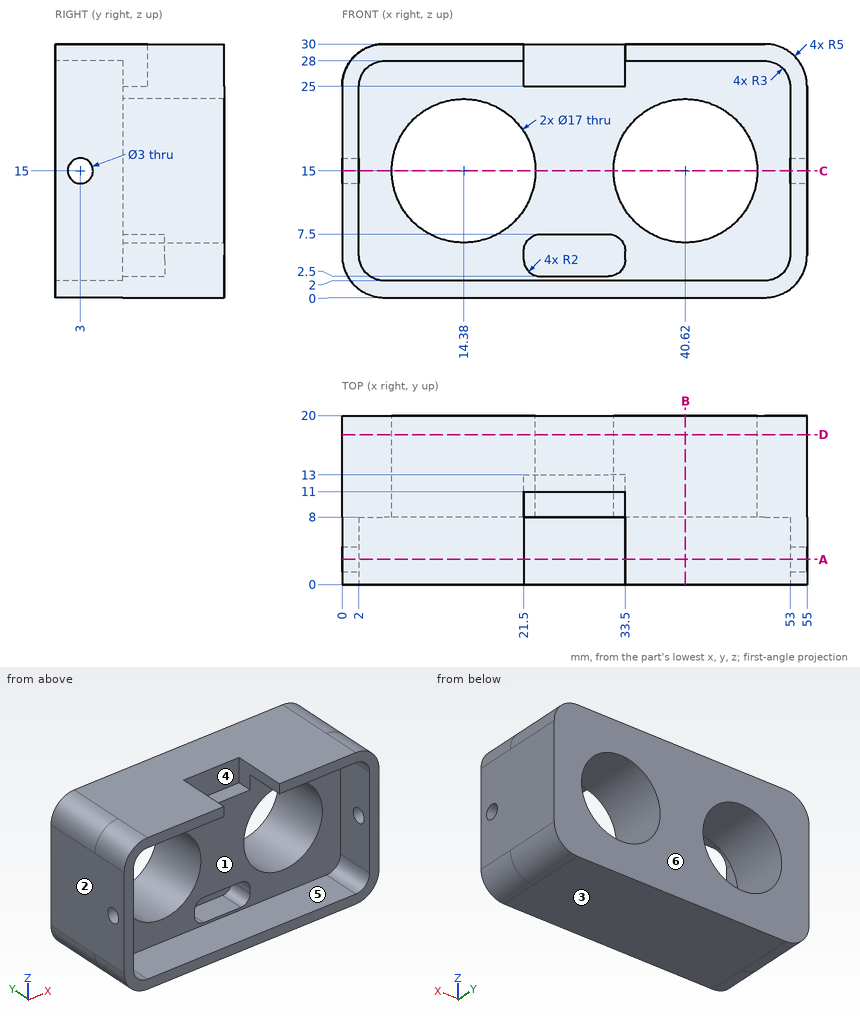
Drawing for the job (mm, zero at the part's lowest x, y, z). A direction names the side the tool comes from. Round coordinates to 2 decimals unless told otherwise and drop trailing zeros. Write each loop counter-clockwise with the first axis right and the second up, starting at its lowest first coordinate (ties: lowest second). Pieces come first, ordered by that corner, then holes. Notation, with made-up numbers: M 42,-9.5 L 72,-9.5 A30 cw 72,13.5 Z; hole C -39.5,85.5 d7. An arc over 180 degrees is marked long. Answer as a JSON object with one key per item and string values. Group by question number.
(1) Cut at D-D (y = 17.75). Give the cut face in (x, z).
(2) Which spindle directions (+Z, -Z, +X, -X, +Y, -Y) get a long thin tool onto all of the face, cutting with end or side? Do the marked faces 4, 5 and 6. Say none if no direction does.
(3) Mould opens along Z. For the marked faces 1, 2 and 3 say: pulls with the +Z half, pulls with the -Z half, needs draft (parallel to the pull), parting line crosses it, or undercut.
(4) Cut at B-B (x = 40.62). Give the cut face in (y, z).
(5) Flat gauge pins, fed straight in: pin 1 (1.5 mm diameter, centred on x = 28.5, z = 6, fed in from -Y); pin 2 (6 mm diameter, centred on x = 22.5, z = 14, fed in from -Y); pin 3 (2.5 mm diameter, centred on x = 26, y = 9.5, fed in from +Z); pin 4 (15.5 mm diameter, centred on x = 40.62, z = 15, fed in from -Y). Where does each tip first touch, or does it go through?
(6) Cut at C-C (z = 15). Give the cut face in (x, y), and give its area (3 significant figures).
(7) Drill centre lines: L1, parallel to X at y = 2, z = 7.5; L2, parallel to X at y = 11.5, z = 15; L3, parallel to X at y = 17.25, z = 14. Where is each one in solid material? Low to high.
(8) Cut at A-A (y = 3). Give the cut face in (x, z), and give its area (3 significant figures).
Responses:
{
 "1": {"outline": "M 0,5 A5 ccw 5,0 L 50,0 A5 ccw 55,5 L 55,25 A5 ccw 50,30 L 5,30 A5 ccw 0,25 Z; hole C 14.38,15 d17; hole C 40.62,15 d17"},
 "2": {"face 4": "+Z, -Y", "face 5": "-Y", "face 6": "+Z, -Z, +X, -X, +Y"},
 "3": {"face 1": "undercut", "face 2": "needs draft", "face 3": "pulls with the -Z half"},
 "4": {"outline": "M 0,0 L 20,0 L 20,6.5 L 8,6.5 L 8,2 L 0,2 Z; M 0,28 L 8,28 L 8,23.5 L 20,23.5 L 20,30 L 0,30 Z"},
 "5": {"pin 1": "stops at y = 13", "pin 2": "stops at y = 8", "pin 3": "stops at z = 25", "pin 4": "passes through"},
 "6": {"outline": "M 0,0 L 2,0 L 2,1.5 L 0,1.5 Z; M 0,4.5 L 2,4.5 L 2,8 L 5.88,8 L 5.88,20 L 0,20 Z; M 22.88,8 L 32.12,8 L 32.12,20 L 22.88,20 Z; M 49.12,8 L 53,8 L 53,4.5 L 55,4.5 L 55,20 L 49.12,20 Z; M 53,0 L 55,0 L 55,1.5 L 53,1.5 Z", "area": "272 mm2"},
 "7": {"L1": "x = 0 to 2, 53 to 55", "L2": "x = 0 to 5.88, 22.88 to 32.12, 49.12 to 55", "L3": "x = 0 to 5.94, 22.82 to 32.18, 49.06 to 55"},
 "8": {"outline": "M 0,5 A5 ccw 5,0 L 50,0 A5 ccw 55,5 L 55,13.5 L 53,13.5 L 53,5 A3 cw 50,2 L 5,2 A3 cw 2,5 L 2,13.5 L 0,13.5 Z; M 0,16.5 L 2,16.5 L 2,25 A3 cw 5,28 L 21.5,28 L 21.5,30 L 5,30 A5 ccw 0,25 Z; M 33.5,28 L 50,28 A3 cw 53,25 L 53,16.5 L 55,16.5 L 55,25 A5 ccw 50,30 L 33.5,30 Z", "area": "274 mm2"}
}
